from build123d import *

# Parameters (mm, degrees)
SKETCH012_R     = 3
PAD005_DEPTH    = 3
SKETCH013_R     = 7.773503
SKETCH013_R_2   = 3
PAD006_DEPTH    = 12.5
POCKET005_DEPTH = 2.5
POCKET006_DEPTH = 5
SKETCH016_R     = 1.5
SKETCH016_W     = 16.799735
SKETCH016_H     = 14
POCKET007_DEPTH = 10
FILLET_R        = 2


with BuildPart() as part:
    # Sketch012 → Pad005 (new body, symmetric)
    with BuildSketch(Plane.XZ):
        with BuildLine():
            ThreePointArc((-15, 5), (-20, 0), (-15, -5))
            Line((-15, -5), (9.047913, -5))
            ThreePointArc((9.047913, -5), (22.773503, 0), (9.047913, 5))
            Line((-15, 5), (9.047913, 5))
        make_face()
        with Locations((15, 0)):
            Circle(SKETCH012_R, mode=Mode.SUBTRACT)
        with BuildLine():
            ThreePointArc((-2.989565, -0.25), (0, -3), (2.989565, -0.25))
            Line((2.989565, -0.25), (7.5, -0.25))
            ThreePointArc((7.5, -0.25), (7.75, 0), (7.5, 0.25))
            Line((2.989565, 0.25), (7.5, 0.25))
            ThreePointArc((2.989565, 0.25), (0, 3), (-2.989565, 0.25))
            Line((-7.5, 0.25), (-2.989565, 0.25))
            ThreePointArc((-7.5, 0.25), (-7.75, 0), (-7.5, -0.25))
            Line((-7.5, -0.25), (-2.989565, -0.25))
        make_face(mode=Mode.SUBTRACT)
        with BuildLine():
            ThreePointArc((-16.5, 3.05), (-19.55, 0), (-16.5, -3.05))
            Line((-16.5, -3.05), (-13.5, -3.05))
            ThreePointArc((-13.5, -3.05), (-10.45, 0), (-13.5, 3.05))
            Line((-16.5, 3.05), (-13.5, 3.05))
        make_face(mode=Mode.SUBTRACT)
    extrude(amount=PAD005_DEPTH, both=True)

    # Sketch013 → Pad006 (join, symmetric)
    with BuildSketch(Plane.XZ):
        with Locations((15, 0)):
            Circle(SKETCH013_R)
        with Locations((15, 0)):
            Circle(SKETCH013_R_2, mode=Mode.SUBTRACT)
    extrude(amount=PAD006_DEPTH, both=True)

    # Sketch014 → Pocket005 (cut, symmetric)
    with BuildSketch(Plane.XZ.offset(11.5)):
        Polygon((17.886751, -5), (20.773503, 0), (17.886751, 5), (12.113249, 5), (9.226497, 0), (12.113249, -5), align=None)
    extrude(amount=POCKET005_DEPTH, both=True, mode=Mode.SUBTRACT)

    # Sketch015 → Pocket006 (cut)
    with BuildSketch(Plane.XZ.offset(-9)):
        Polygon((17.886751, -5), (18.660254, -3.660254), (20, -2.886751), (20, -1.339746), (20.773503, 0), (20, 1.339746), (20, 2.886751), (18.660254, 3.660254), (17.886751, 5), (16.339746, 5), (15, 5.773503), (13.660254, 5), (12.113249, 5), (11.339746, 3.660254), (10, 2.886751), (10, 1.339746), (9.226497, 0), (10, -1.339746), (10, -2.886751), (11.339746, -3.660254), (12.113249, -5), (13.660254, -5), (15, -5.773503), (16.339746, -5), align=None)
    extrude(amount=-POCKET006_DEPTH, mode=Mode.SUBTRACT)

    # Sketch016 → Pocket007 (cut, symmetric)
    with BuildSketch(Plane.XY):
        with Locations((-5, 0)):
            Circle(SKETCH016_R)
        with Locations((5, 0)):
            Circle(SKETCH016_R)
        with Locations((18.475649, 0)):
            Rectangle(SKETCH016_W, SKETCH016_H)
    extrude(amount=POCKET007_DEPTH, both=True, mode=Mode.SUBTRACT)

    # Fillet
    fillet_edges = [part.edges().sort_by_distance(p)[0] for p in [
        (10.075782, -7, 0),
        (10.075782, 7, 0),
    ]]
    fillet(fillet_edges, radius=FILLET_R)


with BuildPart() as part_1:
    # Body022 placement: moved
    add(part.part.moved(Location((0, 47.5, 0))))


solid = part_1.part
Geometry: final body of the model. Coordinates: model frame, mm. A direction names the side the tool comes from. Give positions to 0.01 mm unless a question says otherwise; leave off trailing zeros. Loops run counter-clockwise (first coordinate to the right, second up) from the corner with the lowest first, then second, coordinate; pieces in that order, holes last. Notation, with made-up numbers: (72.25, 85) - (95.25, 85) arc R27 ccw to (95.25, 108) - close; hole circle Ø6 at (14, -23). An arc over 180 degrees is marked (long way). Answer as CSV lines item,"result". Start each with the question number.
1. Section C-C, the plane x = 5. Return loops of the section in (y, z), plus the area to 3 significant figures.
2. Section D-D, the plane y = 48. Give the number of separate pieces and of enclosed holes in the cut face, plus the area to 3 significant figures.
3. Reachability of faces 1 (the face through (-6, 46, -0.25)), 2 (the face through (19.35, 36.726, 2.465)), 3 (the face through (10.65, 53.9, 3.89)), 4 (the face through (9.62, 58.23, 0.68)) from +Z, -Z, +X, -X, +Y, -Y: full face, straight path, thin tool, end or side. Return the list, or none.
4. Pin query (flat end, axial travel): P1, Ø3.5, axis at x = -5, y = 47.5, coming from the -Z side; P2, Ø1.2, axis at y = 58.5, z = -2.5, coming from the -X side; P3, Ø3, axis at x = -10, z = 0.5, coming from the -Y side; P4, Ø1.5, axis at x = -4.5, y = 53, coming from the -Z side. Return the tip coordinate at first contact, or that it passes through.
5. Ray query, L1, parallel to Y at x = -5, z = -2.9; L2, parallel to X at y = 46.25, z = -3.5; L3, parallel to X at y = 47.5, z = 3.25. Return the intervals inside material, ascending.
6. Section B-B, the plane y = 38. Return loops of the section in (x, z), plus the area to 3 significant figures.
7. Section A-A, the plane x = -7. Return loops of the section in (y, z), plus the area to 3 significant figures.
8. Draft query along Z for faces 5 (the face through (-20, 47, 0)), 6 (the face through (15, 37, -5)), 7 (the face through (10.076, 47, 0)). Return one class per face: released by +Z, released by -Z, zero draft, split by the parting line, or undercut.
Answers:
1,outline,"(44.5, -5) - (46, -5) - (46, -0.25) - (44.5, -0.25) - close; (44.5, 0.25) - (46, 0.25) - (46, 5) - (44.5, 5) - close; (49, -5) - (50.5, -5) - (50.5, -0.25) - (49, -0.25) - close; (49, 0.25) - (50.5, 0.25) - (50.5, 5) - (49, 5) - close"
1,area,"28.5 mm2"
2,separate pieces,"4"
2,enclosed holes,"1"
2,area,"157 mm2"
3,face 1,"+Y, -Y"
3,face 2,"-Y"
3,face 3,"+Z, -Z, +X"
3,face 4,"+Y"
4,P1,"stops at z = -5"
4,P2,"stops at x = 7.46"
4,P3,"stops at y = 44.5"
4,P4,"passes through"
5,L1,"y = 44.5 to 46, 49 to 50.5"
5,L2,"x = -18.57 to -5.83, -4.17 to 4.17, 5.83 to 10.08"
5,L3,"x = -18.8 to -6.5, -3.5 to 3.5, 6.5 to 10.08"
6,outline,"circle Ø15.55 at (15, 0); hole (9.23, 0) - (12.11, -5) - (17.89, -5) - (20.77, 0) - (17.89, 5) - (12.11, 5) - close"
6,area,"103 mm2"
7,outline,"(44.5, -5) - (50.5, -5) - (50.5, -0.25) - (44.5, -0.25) - close; (44.5, 0.25) - (50.5, 0.25) - (50.5, 5) - (44.5, 5) - close"
7,area,"57.0 mm2"
8,face 5,"split by the parting line"
8,face 6,"undercut"
8,face 7,"zero draft"
